```python
from build123d import *

# Parameters (mm, degrees)
SKETCH_1_W      = 5
SKETCH_1_H      = 20
SKETCH_1_W_2    = 45
SKETCH_1_H_2    = 5
SKETCH_1_H_3    = 25
SKETCH_1_W_3    = 30
EXTRUDE_1_DEPTH = 150


with BuildPart() as part:
    # Sketch 1 → Extrude 1 (new body)
    with BuildSketch(Plane(origin=(0, 0, 0), x_dir=(0, 0, -1), z_dir=(1, 0, 0))):
        with Locations((32.5, 15)):
            Rectangle(SKETCH_1_W, SKETCH_1_H)
        with Locations((22.5, 2.5)):
            Rectangle(SKETCH_1_W_2, SKETCH_1_H_2)
        with Locations((2.5, 17.5)):
            Rectangle(SKETCH_1_W, SKETCH_1_H_3)
        with Locations((30, 27.5)):
            Rectangle(SKETCH_1_W_3, SKETCH_1_H_2)
    extrude(amount=EXTRUDE_1_DEPTH)


solid = part.part
```
Input: part model. Units: mm. Frame: model coordinates. A direction names the side the tool comes from. Give positions to 0.01 mm unless a question says otherwise; leave off trailing zeros. Order: outer loops, then holes, each group sorted by start corner. A loop starts at its lowest first (then second) coordinate and runs counter-clockwise, first axis right, second up.
1. Reachability of faces 5 (the flat face through (74, 17, -5)), 6 (the flat face through (74, 25, -40)), 7 (the flat face through (74, 5, -17)), 8 (the flat face through (74, 15, 0)), 9 (the flat face through (150, 25.2, -22.2)) from +Z, -Z, +X, -X, +Y, -Y: full face, straight path, thin tool, end or side. Return the list, or none.
Derived:
face 5: +X, -X, +Y
face 6: -Z, +X, -X
face 7: +X, -X
face 8: +Z, +X, -X, +Y, -Y
face 9: +Z, -Z, +X, +Y, -Y
2. Material intervals for L1, parallel to Y at x = 23, z = -17.5; L2, parallel to Z at x = 28, y = 27.75; L3, parallel to Z at x = 65, y = 14, sorted ascending.
Derived:
L1: y = 0 to 5, 25 to 30
L2: z = -45 to -15, -5 to 0
L3: z = -35 to -30, -5 to 0
3. Section A-A on y = 18. Return the cut outline in (x, z).
Derived:
outline: (0, -35) - (150, -35) - (150, -30) - (0, -30) - close; (0, -5) - (150, -5) - (150, 0) - (0, 0) - close
4. Section D-D on z = -11. Return the cut outline in (x, y).
Derived:
outline: (0, 0) - (150, 0) - (150, 5) - (0, 5) - close
5. Section C-C on x = 78. Return the cut outline in (y, z), and give its area (3 significant figures).
Derived:
outline: (0, -45) - (5, -45) - (5, -35) - (25, -35) - (25, -45) - (30, -45) - (30, -15) - (25, -15) - (25, -30) - (5, -30) - (5, -5) - (30, -5) - (30, 0) - (0, 0) - close
area: 600 mm2
6. Section B-B on z = -22.5. Return the cut outline in (x, y), and give its area (3 significant figures).
Derived:
outline: (0, 0) - (150, 0) - (150, 5) - (0, 5) - close; (0, 25) - (150, 25) - (150, 30) - (0, 30) - close
area: 1,500 mm2
7. Pin query (flat end, axial travel): pin 1 (2 mm diameter, centred on y = 6.5, z = -14, fed in from -X); pin 2 (8 mm diameter, centred on x = 46.5, z = -23.5, fed in from -Y); pin 3 (6 mm diameter, centred on x = 109.5, y = 11, fed in from -Z). Return the tip coordinate at first contact, or that it passes through.
Derived:
pin 1: passes through
pin 2: stops at y = 0
pin 3: stops at z = -35
8. Mould query, pull axis Y, two halves, no side actions, for faces 1 (the flat face through (74, 27, -45)), 2 (the flat face through (74, 30, -2)), 3 (the flat face through (74, 25, -22)), 4 (the flat face through (74, 15, -35)). Classes: released by +Y, released by -Y, zero draft, split by the parting line, or undercut.
Derived:
face 1: zero draft
face 2: released by +Y
face 3: undercut
face 4: undercut
